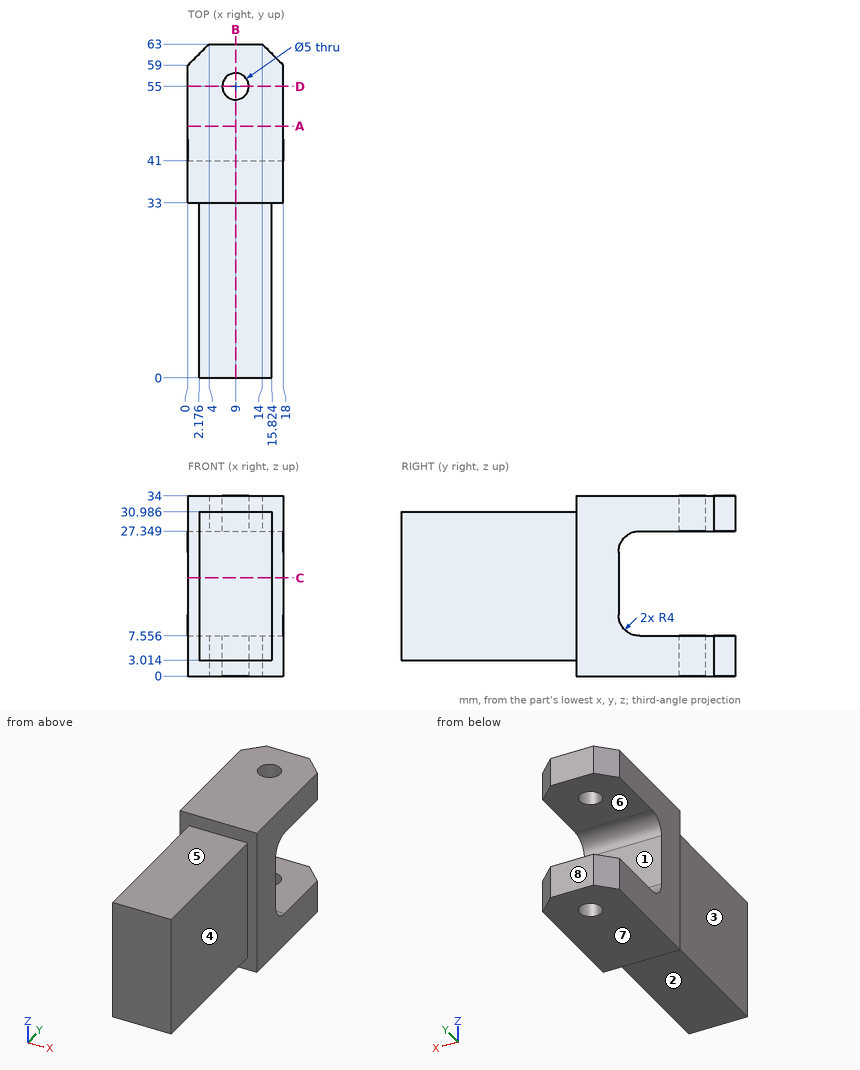
The drawing under review shows one solid part. Ordinate dimensions are in mm from its lowest x, y, z. A direction names the side the tool comes from. Round coordinates to 2 decimals unless told otherwise and drop trailing zeros. Write each loop counter-clockwise with the first axis right and the second up, starting at its lowest first coordinate (ties: lowest second). Pieces come first, ordered by that corner, then holes. Notation, with made-up numbers: M 40,87.5 L 87,87.5 A8 cw 87,91.5 Z; hole C 53.5,-12 d5. An arc over 180 degrees is marked long. One line per item, written item: value. Start each with the question number.
(1) Wall thickness on line 1 (Y direction, x = 9, z = 4.75); line 2 (Y direction, x = 9, z = 1.5); line 3 (Y direction, x = 8, z = 17): over which ranges is each line inside the solid? List them lowest first.
(2) Insertion check: pin 1 (9 mm diameter, centred on x = 11, z = 24.5, fed in from -Y); pin 2 (3 mm diameter, centred on x = 9, y = 55, fed in from +Z); pin 3 (8.5 mm diameter, centred on y = 20, z = 23.5, fed in from +X); pin 4 (4 mm diameter, centred on x = 11.5, y = 21, fed in from +Z). Each pin has a flat end and moves straight along its axis. Give the tip position at first contact, or say it passes through.
(3) We need section D-D (y = 55). Give the boundary of the cut face in (x, z), and give its area (3 significant figures).
(4) We need section B-B (x = 9). Give the boundary of the cut face in (y, z).
(5) Machinability: for the marked faces 1, 2, 3 and 4, which of the approach directions +Z, -Z, +X, -X, +Y, -Y give a long, thin tool a straight path to every point of the face, cutting with its end or side? Answer none if there is none.
(6) We need section C-C (z = 18.5). Give the boundary of the cut face in (x, y).
(7) The part is to be moulded in two halves that separate along Z. For the marked faces 5, 6, 7 and 8, say which applies: released by +Z, released by -Z, zero draft, split by the parting line, or undercut.
(8) We need section A-A (y = 47.5). Give the boundary of the cut face in (x, z).
Result:
1. line 1: 0 to 52.5, 57.5 to 63
1. line 2: 33 to 52.5, 57.5 to 63
1. line 3: 0 to 41
2. pin 1: y = 0
2. pin 2: through
2. pin 3: x = 15.82
2. pin 4: z = 30.99
3. outline: M 0,0 L 6.5,0 L 6.5,7.56 L 0,7.56 Z; M 0,27.35 L 6.5,27.35 L 6.5,34 L 0,34 Z; M 11.5,0 L 18,0 L 18,7.56 L 11.5,7.56 Z; M 11.5,27.35 L 18,27.35 L 18,34 L 11.5,34 Z
3. area: 185 mm²
4. outline: M 0,3.01 L 33,3.01 L 33,0 L 52.5,0 L 52.5,7.56 L 45,7.56 A4 cw 41,11.56 L 41,23.35 A4 cw 45,27.35 L 52.5,27.35 L 52.5,34 L 33,34 L 33,30.99 L 0,30.99 Z; M 57.5,0 L 63,0 L 63,7.56 L 57.5,7.56 Z; M 57.5,27.35 L 63,27.35 L 63,34 L 57.5,34 Z
5. face 1: +X, -X, +Y
5. face 2: -Z, +X, -X, -Y
5. face 3: +Z, -Z, -X, -Y
5. face 4: +Z, -Z, +X, -Y
6. outline: M 0,33 L 2.18,33 L 2.18,0 L 15.82,0 L 15.82,33 L 18,33 L 18,41 L 0,41 Z
7. face 5: released by +Z
7. face 6: undercut
7. face 7: released by -Z
7. face 8: zero draft
8. outline: M 0,0 L 18,0 L 18,7.56 L 0,7.56 Z; M 0,27.35 L 18,27.35 L 18,34 L 0,34 Z
